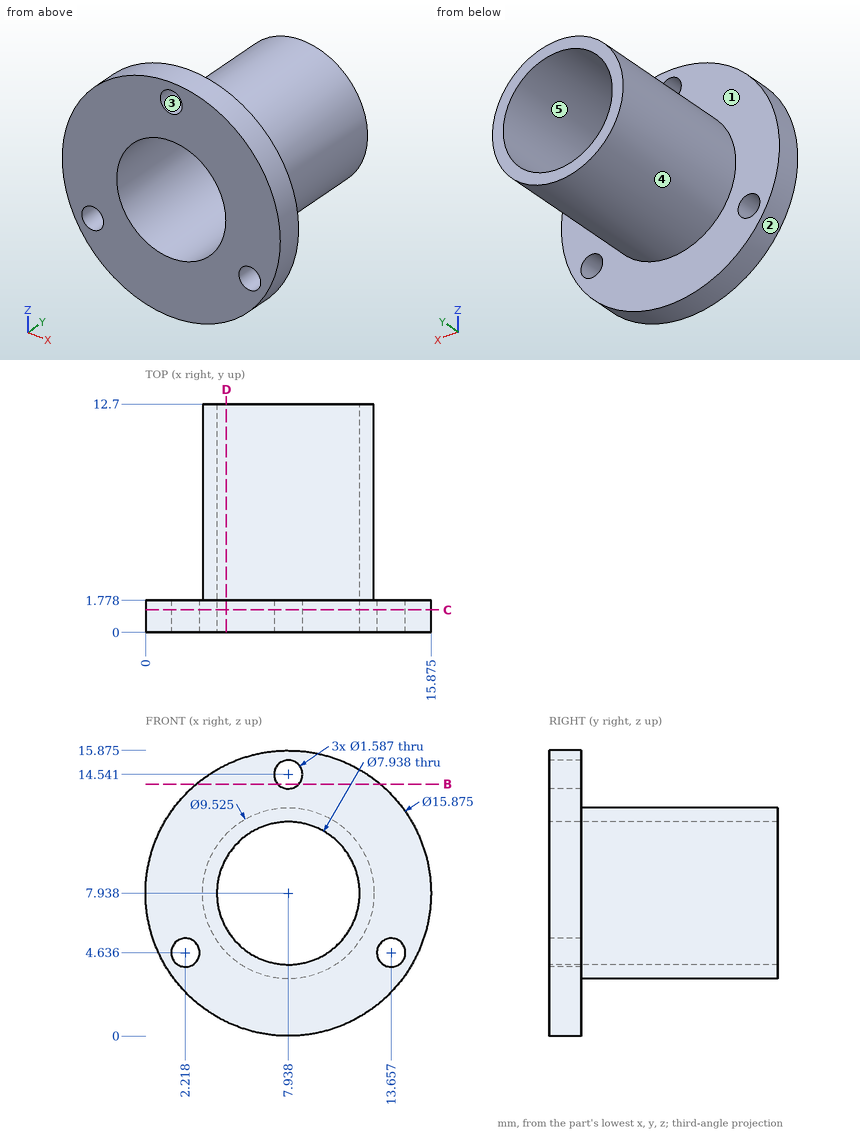
Could you check a few things on this drawing? It's one solid part, dimensions in mm from its lowest x, y, z. A direction names the side the tool comes from. Give positions to 0.01 mm unless a question says otherwise; leave off trailing zeros. Order: outer loops, then holes, each group sorted by start corner. A loop starts at its lowest first (then second) coordinate and runs counter-clockwise, first axis right, second up. Notation, with made-up numbers: (86.25, -1.75) - (92.25, -1.75) arc R27 ccw to (92.25, 36.25) - close; hole circle Ø8 at (31.25, -23.5). An arc over 180 degrees is marked (long way). Return JSON: item names as keys, results as strings. Group by question number.
Q1. Suppose I cut it at D-D, the plane x = 4.5. Please give me the cut outline in (y, z).
Q2. Please list where these lines run through material, in increasing order: line 1 along X through (y, z) = (9.75, 8) (1 decimal); line 2 along X through (y, z) = (10, 6.5) (1 decimal); line 3 along Y through (x, z) = (2.5, 9.5). Write a range as [from, to].
Q3. Suppose I cut it at B-B, the plane z = 14. Please give me the cut outline in (x, y) (1 decimal).
Q4. Suppose I cut it at C-C, the plane y = 1.25. State how many separate pieces and enclosed holes the cut face has.
Q5. Which directions (+Z, -Z, +X, -X, +Y, -Y) give clear straight access to the entire face, cutting with the end or side of a thin tool? Please do the marked faces 4 and 5.
Q6. Thinking about a two-plate mould opening in Z: for the marked faces 1, 2 and 3, which applies, pulls with the +Z half, pulls with the -Z half, needs draft (parallel to the pull), parting line crosses it, or undercut?
Q7. Will these pins go through, and if not, where does the flat tip stop? pin 1 Ø4 at (y, z) = (8.5, 8) entering from -X (1 decimal); pin 2 Ø2 at (y, z) = (9, 6) entering from +X; pin 3 Ø6 at (x, y) = (13.5, 3.5) entering from -Z; pin 4 Ø1.3 at (x, z) = (7.94, 14.54) entering from -Y.
Resolved:
{
 "1": {"outline": "(0, 0.78) - (1.78, 0.78) - (1.78, 4.64) - (12.7, 4.64) - (12.7, 5.95) - (0, 5.95) - close; (0, 9.92) - (12.7, 9.92) - (12.7, 11.23) - (1.78, 11.23) - (1.78, 15.09) - (0, 15.09) - close"},
 "2": {"line 1": "x = [3.2, 4], [11.9, 12.7]", "line 2": "x = [3.4, 4.2], [11.6, 12.5]", "line 3": "y = [0, 1.78]"},
 "3": {"outline": "(2.8, 0) - (7.4, 0) - (7.4, 1.8) - (2.8, 1.8) - close; (8.5, 0) - (13.1, 0) - (13.1, 1.8) - (8.5, 1.8) - close"},
 "4": {"separate pieces": "1", "enclosed holes": "4"},
 "5": {"face 4": "+Y", "face 5": "+Y, -Y"},
 "6": {"face 1": "needs draft", "face 2": "parting line crosses it", "face 3": "undercut"},
 "7": {"pin 1": "stops at x = 3.2", "pin 2": "stops at x = 12.61", "pin 3": "stops at z = 0.63", "pin 4": "passes through"}
}
